```python
from build123d import *

# Parameters (mm, degrees)
SKETCH_1_W          = 41.5
SKETCH_1_H          = 20
SKETCH_2_R          = 6
CUT_EXTRUDE_1_DEPTH = 20
SKETCH_2_3_R        = 6
CUT_EXTRUDE_2_DEPTH = 20


with BuildPart() as part:
    # Sketch 1 → Revolve 1 (revolve)
    with BuildSketch(Plane.XY, mode=Mode.PRIVATE) as revolve_1_sk:
        with Locations((33.25, 10)):
            Rectangle(SKETCH_1_W, SKETCH_1_H)
    revolve(revolve_1_sk.sketch.rotate(Axis((0, 0, 0), (0, 1, 0)), 90), axis=Axis((0, 0, 0), (0, 1, 0)))

    # Sketch 2 → Cut-Extrude 1 (cut)
    with BuildSketch(Plane(origin=(0, 20, 0), x_dir=(1, 0, 0), z_dir=(0, 1, 0))):
        with Locations(Location((0, 26, 0), (0, 0, 270))):
            Circle(SKETCH_2_R)
    extrude(amount=-CUT_EXTRUDE_1_DEPTH, mode=Mode.SUBTRACT)

    # Sketch 2_3 → Cut-Extrude 2 (cut)
    with BuildSketch(Plane(origin=(0, 20, 0), x_dir=(1, 0, 0), z_dir=(0, 1, 0))):
        with Locations(Location((0, 26, 0), (0, 0, 270))):
            Circle(SKETCH_2_3_R)
        with Locations(Location((0, -26, 0), (0, 0, 270))):
            Circle(SKETCH_2_3_R)
        with BuildLine():
            Line((-11.842719282, 4), (-15.6, 4))
            Line((-15.6, 4), (-15.6, -4))
            Line((-15.6, -4), (-11.842719282, -4))
            ThreePointArc((-11.842719282, -4), (12.5, 0), (-11.842719282, 4))
        make_face()
    extrude(amount=-CUT_EXTRUDE_2_DEPTH, mode=Mode.SUBTRACT)


solid = part.part
```
Can you work these out from the model? Positions are in its coordinate system, mm. A direction names the side the tool comes from. Coordinates: 2 decimals unless noted, no trailing zeros. Write each loop counter-clockwise with the first axis right and the second up, starting at its lowest first coordinate (ties: lowest second). Pieces come first, ordered by that corner, then holes. Notation, with made-up numbers: (73.25, -25.5) - (87.25, -25.5) arc R18 ccw to (87.25, -13.5) - close; hole circle Ø2 at (84, 32). An arc over 180 degrees is marked (long way). Return JSON: item names as keys, results as strings.
Q1. If we section it at D-D (z = 23): Please give me the cut outline in (x, y).
Computed values:
{"outline": "(-48.86, 0) - (-5.2, 0) - (-5.2, 20) - (-48.86, 20) - close; (5.2, 0) - (48.86, 0) - (48.86, 20) - (5.2, 20) - close"}
Q2. Thinking about a two-plate mould opening in X: for faces 1 (the flat face through (-1, 20, -13)), 2 (the cylindrical face through (0, 10, -32)), 3 (the cylindrical face through (52.716, 10.14, 11.706)), 4 (the flat face through (-14, 10, -4)), which applies, +X half, -X half, draft (parallel to the pull), parting line (faces both ways), or undercut?
Computed values:
{"face 1": "draft", "face 2": "undercut", "face 3": "parting line", "face 4": "undercut"}
Q3. I'm going to push flat-ended pins straight in: pin 1 Ø2.5 at (y, z) = (9, -1.5) entering from +X; pin 2 Ø6 at (x, z) = (-30.5, -17.5) entering from -Y; pin 3 Ø10 at (y, z) = (8.5, -25) entering from -X; pin 4 Ø1.5 at (x, z) = (6.5, 7.5) entering from +Y. Where does each tip first touch, or does it pass through?
Computed values:
{"pin 1": "stops at x = 54", "pin 2": "stops at y = 0", "pin 3": "stops at x = -50.16", "pin 4": "passes through"}
Q4. If we section it at A-A (z = 0): Please give me the cut outline in (x, y), then the cut area to 3 significant figures.
Computed values:
{"outline": "(-54, 0) - (-15.6, 0) - (-15.6, 20) - (-54, 20) - close; (12.5, 0) - (54, 0) - (54, 20) - (12.5, 20) - close", "area": "1,600 mm2"}
Q5. Please list where these lines run through material, in increasing order: L1, parallel to X at y = 8, z = 0; L2, parallel to Z at x = 43.5, y = 3.5; L3, parallel to X at y = 13.75, z = -26. Write a range as from..to.
Computed values:
{"L1": "x = -54..-15.6, 12.5..54", "L2": "z = -32..32", "L3": "x = -47.33..-6, 6..47.33"}
Q6. If we section it at B-B (y = 13): Please give me the cut outline in (x, z).
Computed values:
{"outline": "circle Ø108 at (0, 0); hole (-15.6, -4) - (-11.84, -4) arc R12.5 ccw (long way) to (-11.84, 4) - (-15.6, 4) - close; hole circle Ø12 at (0, -26); hole circle Ø12 at (0, 26)"}
Q7. On a 3-axis mill with a long thin cutter (end or side, diameter ignored), from which of +Z, -Z, +X, -X, +Y, -Y can I reach the whole of each face in a straight line? I mean faces 5 (the flat face through (-1, 0, -13)), 6 (the flat face through (-15.6, 10, 0)). Say none if no direction works.
Computed values:
{"face 5": "+Z, -Z, +X, -X, -Y", "face 6": "+Y, -Y"}
Q8. If we section it at C-C (x = 0): Please give me the cut outline in (y, z), then the cut area to 3 significant figures.
Computed values:
{"outline": "(0, -54) - (20, -54) - (20, -32) - (0, -32) - close; (0, -20) - (20, -20) - (20, -12.5) - (0, -12.5) - close; (0, 12.5) - (20, 12.5) - (20, 20) - (0, 20) - close; (0, 32) - (20, 32) - (20, 54) - (0, 54) - close", "area": "1,180 mm2"}
